```python
from build123d import *

# Parameters (mm, degrees)
SKETCH1_W           = 571.5
SKETCH1_H           = 889
BOSS_EXTRUDE1_DEPTH = 19.05
SKETCH2_W           = 257.175
SKETCH2_H           = 850.9
CUT_EXTRUDE1_DEPTH  = 20.05


with BuildPart() as part:
    # Sketch1 → Boss-Extrude1 (new body)
    with BuildSketch(Plane.XY):
        Rectangle(SKETCH1_W, SKETCH1_H)
    extrude(amount=-BOSS_EXTRUDE1_DEPTH)

    # Sketch2 → Cut-Extrude1 (cut, through all)
    with BuildSketch(Plane.XY):
        with Locations((-138.1125, 0)):
            Rectangle(SKETCH2_W, SKETCH2_H)
        with Locations((138.1125, 0)):
            Rectangle(SKETCH2_W, SKETCH2_H)
    extrude(amount=-CUT_EXTRUDE1_DEPTH, mode=Mode.SUBTRACT)


solid = part.part
```
Geometry: final body of the model. Coordinates: model frame, mm. A direction names the side the tool comes from. Round coordinates to 2 decimals unless told otherwise and drop trailing zeros. Order: outer loops, then holes, each group sorted by start corner. A loop starts at its lowest first (then second) coordinate and runs counter-clockwise, first axis right, second up. Notation, with made-up numbers: (10.5, 61) - (46.5, 61) arc R13 ccw to (46.5, 81) - close; hole circle Ø2 at (69, 51.5). An arc over 180 degrees is marked (long way). Use CSV: the item, a comma, the result in double quotes. Start each with the question number.
Q1. Section query A-A (y = -335.5). Return loops of the section in (x, z) (3 decimals), and give its area (3 significant figures).
Q2. Material intervals for line 1 along X through (y, z) = (42.5, -15.5) (3 decimals); line 2 along Y through (x, z) = (-109.5, -6.25), sorted ascending. Write a range as from..to.
Q3. Section query B-B (x = -246). Return loops of the section in (y, z).
Q4. Section query C-C (z = -15.25). Return loops of the section in (x, y) (3 decimals).
Q5. Mould query, pull axis Y, two halves, no side actions, for faces 1 (the face through (-140, 425.45, -9)), 2 (the face through (-1, 2, -19.05)), 3 (the face through (-140, -425.45, -9)), 4 (the face through (-4, 444.5, -9)). Classes: +Y half, -Y half, draft (parallel to the pull), parting line (faces both ways), or undercut.
Q6. Access query for faces 5 (the face through (136, 425.45, -9)), 6 (the face through (-4, -444.5, -9)). Directions: +Z, -Z, +X, -X, +Y, -Y. A direction counts if a zero-diameter tool reaches every point of the face in a straight line with its end or side. Return the directions, or none.
Result set:
1,outline,"(-285.75, -19.05) - (-266.7, -19.05) - (-266.7, 0) - (-285.75, 0) - close; (-9.525, -19.05) - (9.525, -19.05) - (9.525, 0) - (-9.525, 0) - close; (266.7, -19.05) - (285.75, -19.05) - (285.75, 0) - (266.7, 0) - close"
1,area,"1,090 mm2"
2,line 1,"x = -285.75..-266.7, -9.525..9.525, 266.7..285.75"
2,line 2,"y = -444.5..-425.45, 425.45..444.5"
3,outline,"(-444.5, -19.05) - (-425.45, -19.05) - (-425.45, 0) - (-444.5, 0) - close; (425.45, -19.05) - (444.5, -19.05) - (444.5, 0) - (425.45, 0) - close"
4,outline,"(-285.75, -444.5) - (285.75, -444.5) - (285.75, 444.5) - (-285.75, 444.5) - close; hole (-266.7, -425.45) - (-9.525, -425.45) - (-9.525, 425.45) - (-266.7, 425.45) - close; hole (9.525, -425.45) - (266.7, -425.45) - (266.7, 425.45) - (9.525, 425.45) - close"
5,face 1,"undercut"
5,face 2,"draft"
5,face 3,"undercut"
5,face 4,"+Y half"
6,face 5,"+Z, -Z"
6,face 6,"+Z, -Z, +X, -X, -Y"
